Design review of the part built by this model. Coordinates are the model's own, in mm. Face numbers are marked on the shaded views. Coordinates: 2 decimals unless noted, no trailing zeros. Write each loop counter-clockwise with the first axis right and the second up, starting at its lowest first coordinate (ties: lowest second). Pieces come first, ordered by that corner, then holes. Notation, with made-up numbers: M -16,71.5 L -5,71.5 A12 ccw -5,84.5 Z; hole C 85.25,74 d7. An arc over 180 degrees is marked long. Write item = value, one per line.
```python
from build123d import *

# Parameters (mm, degrees)
SKETCH1_W           = 60
SKETCH1_H           = 80
SKETCH1_R           = 18.75
BOSS_EXTRUDE1_DEPTH = 25
SKETCH4_R           = 12.4
CUT_EXTRUDE1_DEPTH  = 51.75


with BuildPart() as part:
    # Sketch1 → Boss-Extrude1 (new body, symmetric)
    with BuildSketch(Plane(origin=(0, 0, 0), x_dir=(1, 0, 0), z_dir=(0, 1, 0))):
        with Locations((30, 40)):
            Rectangle(SKETCH1_W, SKETCH1_H)
        with Locations((30, 50.75)):
            Circle(SKETCH1_R, mode=Mode.SUBTRACT)
    extrude(amount=BOSS_EXTRUDE1_DEPTH, both=True)

    # Sketch4 → Cut-Extrude1 (cut, through all)
    with BuildSketch(Plane.XY.offset(-50.75)):
        with Locations((30, 0)):
            Circle(SKETCH4_R)
    extrude(amount=CUT_EXTRUDE1_DEPTH, mode=Mode.SUBTRACT)


solid = part.part
```
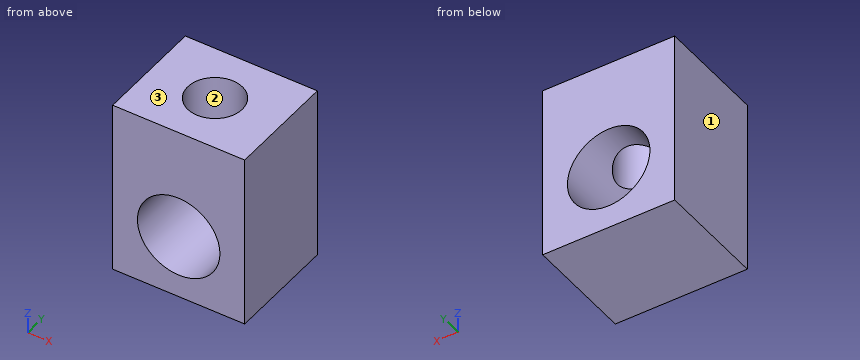
Q1. Consider section B-B, the plane x = 30. State the section outline as (y, z) points, and give its area (3 significant figures).
Check result:
outline = M -25,-80 L 25,-80 L 25,-69.5 L -25,-69.5 Z; M -25,-32 L -12.4,-32 L -12.4,0 L -25,0 Z; M 12.4,-32 L 25,-32 L 25,0 L 12.4,0 Z
area = 1,330 mm²
Q2. Consider section C-C, the plane y = 0. State the section outline as (x, z) points.
Check result:
outline = M 0,-80 L 60,-80 L 60,0 L 42.4,0 L 42.4,-36.69 A18.75 cw long 17.6,-36.69 L 17.6,0 L 0,0 Z
Q3. For P1, Ø22.5, axis at x = 30, z = -50.75, coming from the -Y side, flat-tipped, find the tip position at first contact; note if it passes through.
Check result:
P1 = through
Q4. Consider section A-A, the plane z = -50.75. State the section outline as (x, y) points.
Check result:
outline = M 0,-25 L 11.25,-25 L 11.25,25 L 0,25 Z; M 48.75,-25 L 60,-25 L 60,25 L 48.75,25 Z
Q5. Wall thickness on line 1 (Y direction, x = 30, z = -27); line 2 (X direction, y = -21.5, z = -50) (3 decimals); line 3 (X direction, y = 0, z = -9): over which ranges is each line inside the solid? List them lowest first.
Check result:
line_1 = -25 to -12.4, 12.4 to 25
line_2 = 0 to 11.265, 48.735 to 60
line_3 = 0 to 17.6, 42.4 to 60
Q6. The part is to be moulded in two halves that separate along X. For the marked faces 1, 2 and 3, say which applies: +X half, -X half, draft (parallel to the pull), parting line (faces both ways), or undercut.
Check result:
face_1 = -X half
face_2 = undercut
face_3 = draft
Q7. Consider section D-D, the plane z = -15. State the section outline as (x, y) points.
Check result:
outline = M 0,-25 L 60,-25 L 60,25 L 0,25 Z; hole C 30,0 d24.8
